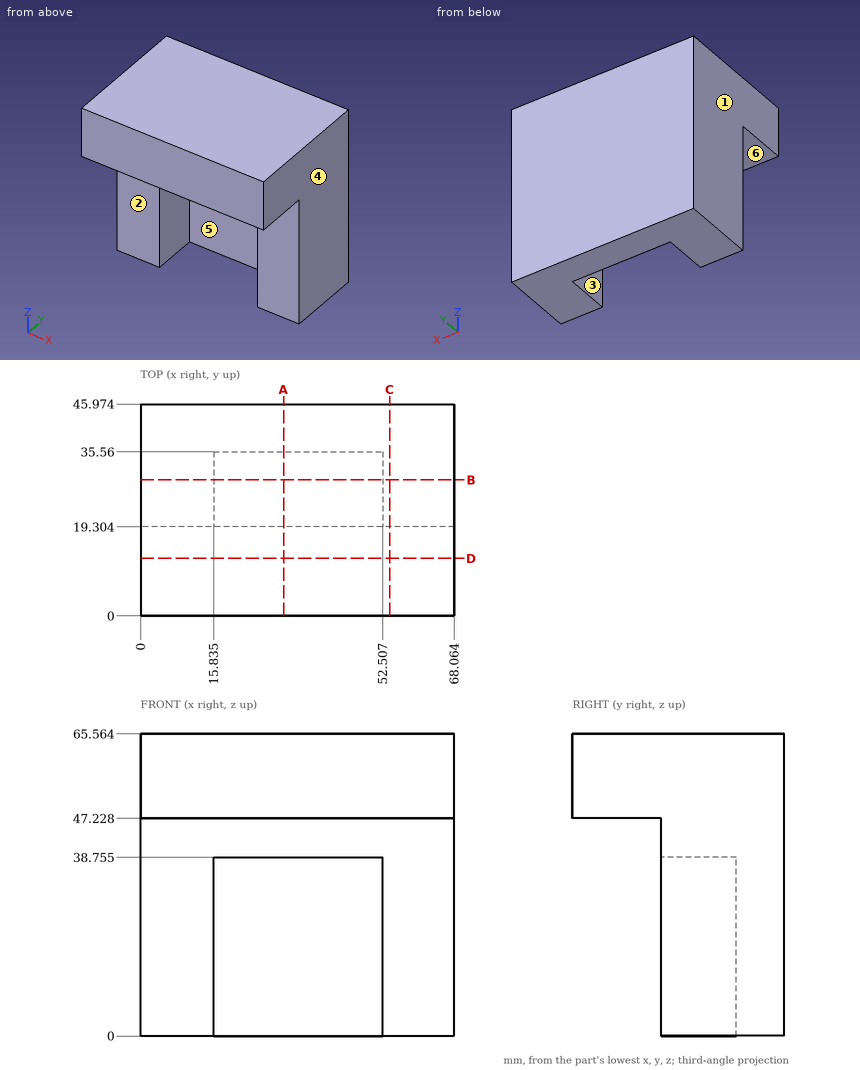
For this review, use the dimensioned drawing (mm, ordinates from the lowest corner) and the shaded views. A direction names the side the tool comes from. Round coordinates to 2 decimals unless told otherwise and drop trailing zeros. Order: outer loops, then holes, each group sorted by start corner. A loop starts at its lowest first (then second) coordinate and runs counter-clockwise, first axis right, second up. Notation, with made-up numbers: (18, 70.25) -> (74, 70.25) arc R32 cw to (74, 97.25) -> close; hole circle Ø5 at (43, -21). An arc over 180 degrees is marked (long way). Write item = value, one per line. Start each with the question number.
Item 1: Consider section D-D on y = 12.5. Write out the cut boundary in (x, z), plus the area to 3 significant figures.
Item 2: Consider section A-A on x = 31. Write out the cut boundary in (y, z) (1 decimal), plus the area to 3 significant figures.
Item 3: Mouldability with a two-part tool opening along X and no side actions: class the marked faces 1, 2 and 3 as released by +X, released by -X, zero draft, split by the parting line, or undercut.
Item 4: Consider section B-B on y = 29.5. Write out the cut boundary in (x, z) (1 decimal).
Item 5: For line 1 along Z through (x, y) = (16, 23) (1 decimal); line 2 along Y through (x, z) = (16.5, 33); line 3 along Z through (x, y) = (16.5, 14.5), list the stretches that pass through material, from the lowest coordinate up.
Item 6: For the marked faces 4, 5 and 6, list the 3-axis set-ups (+Z, -Z, +X, -X, +Y, -Y) from which the entire face can be reached by the end or side of a thin tool; tool diameter is ignored.
Item 7: Consider section C-C on x = 54. Write out the cut boundary in (y, z), plus the area to 3 significant figures.
Item 8: Clearance check with flat-ended pins moving along their axes: pin 1 Ø6 at (x, y) = (42, 31) entering from -Z (1 decimal); pin 2 Ø10 at (x, y) = (23, 12.5) entering from -Z; pin 3 Ø3 at (x, z) = (33, 57.5) entering from -Y; pin 4 Ø6 at (x, z) = (12.5, 33) entering from -Y. State where each tip first meets the part, or that it passes through.
Conclusion:
q1.outline = (0, 47.23) -> (68.06, 47.23) -> (68.06, 65.56) -> (0, 65.56) -> close
q1.area = 1,250 mm2
q2.outline = (0, 47.2) -> (19.3, 47.2) -> (19.3, 38.8) -> (35.6, 38.8) -> (35.6, 0) -> (46, 0) -> (46, 65.6) -> (0, 65.6) -> close
q2.area = 1,470 mm2
q3.face_1 = released by -X
q3.face_2 = zero draft
q3.face_3 = undercut
q4.outline = (0, 0) -> (15.8, 0) -> (15.8, 38.8) -> (52.5, 38.8) -> (52.5, 0) -> (68.1, 0) -> (68.1, 65.6) -> (0, 65.6) -> close
q5.line_1 = 38.8 to 65.6
q5.line_2 = 35.56 to 45.97
q5.line_3 = 47.23 to 65.56
q6.face_4 = +Z, -Z, +X, +Y, -Y
q6.face_5 = -Z, -Y
q6.face_6 = -Z, +X, -X, -Y
q7.outline = (0, 47.23) -> (19.3, 47.23) -> (19.3, 0) -> (45.97, 0) -> (45.97, 65.56) -> (0, 65.56) -> close
q7.area = 2,100 mm2
q8.pin_1 = 38.8
q8.pin_2 = 47.23
q8.pin_3 = 0
q8.pin_4 = 19.3
